Could you check a few things on this drawing? It's one solid part, dimensions in mm from its lowest x, y, z. Coordinates: 2 decimals unless noted, no trailing zeros. Write each loop counter-clockwise with the first axis right and the second up, starting at its lowest first coordinate (ties: lowest second). Pieces come first, ordered by that corner, then holes. Notation, with made-up numbers: M 2.5,-31.5 L 48.5,-31.5 A21 cw 48.5,-16.5 Z; hole C 81,-35 d10. An arc over 180 degrees is marked long. Use a Markdown table: item, result.
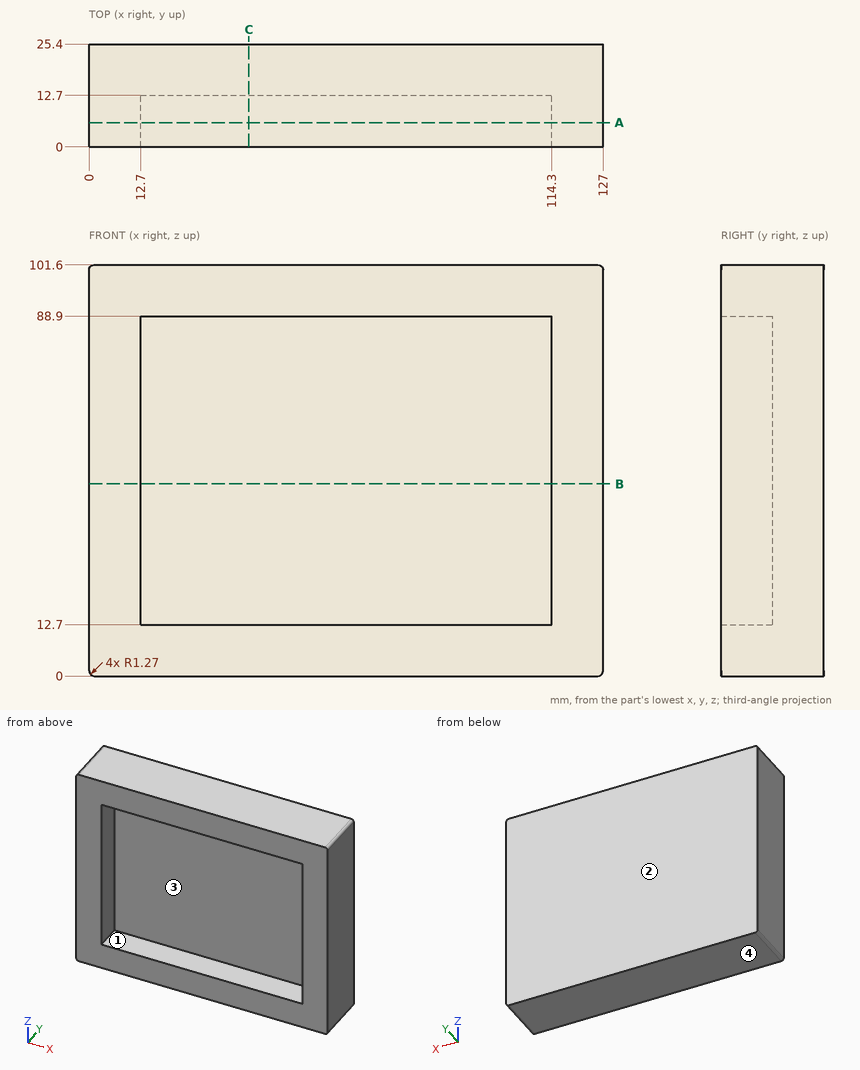
1. Suppose I cut it at A-A on y = 6. Write out the boundary of the cut face in (x, z).
Answers follow:
| item | result |
|---|---|
| outline | M 0,1.27 A1.27 ccw 1.27,0 L 125.73,0 A1.27 ccw 127,1.27 L 127,100.33 A1.27 ccw 125.73,101.6 L 1.27,101.6 A1.27 ccw 0,100.33 Z; hole M 12.7,12.7 L 114.3,12.7 L 114.3,88.9 L 12.7,88.9 Z |
2. Suppose I cut it at B-B on z = 47.5. Write out the boundary of the cut face in (x, y).
Answers follow:
| item | result |
|---|---|
| outline | M 0,0 L 12.7,0 L 12.7,12.7 L 114.3,12.7 L 114.3,0 L 127,0 L 127,25.4 L 0,25.4 Z |
3. We'd pull the mould along Z, two halves only. Please class the marked faces 1, 2, 3 and 4: +Z half, -Z half, draft (parallel to the pull), parting line (faces both ways), or undercut.
Answers follow:
| item | result |
|---|---|
| face 1 | undercut |
| face 2 | draft |
| face 3 | undercut |
| face 4 | -Z half |
4. Suppose I cut it at C-C on x = 39.5. Write out the boundary of the cut face in (y, z).
Answers follow:
| item | result |
|---|---|
| outline | M 0,0 L 25.4,0 L 25.4,101.6 L 0,101.6 L 0,88.9 L 12.7,88.9 L 12.7,12.7 L 0,12.7 Z |
5. I need wall thicknesses on probe 1 along X at (y, z) = (10.75, 13.5); probe 2 along Z at (x, y) = (98, 8.5); probe 3 along Y at (x, z) = (85, 16). Which ranges of each line are inside material? Lowest first, please.
Answers follow:
| item | result |
|---|---|
| probe 1 | x = 0 to 12.7, 114.3 to 127 |
| probe 2 | z = 0 to 12.7, 88.9 to 101.6 |
| probe 3 | y = 12.7 to 25.4 |
6. Will this pin go through, and if not, where does the flat tip stop? pin 1 Ø8 at (x, z) = (56.5, 28) entering from -Y.
Answers follow:
| item | result |
|---|---|
| pin 1 | stops at y = 12.7 |
